Part model, mm, in its own coordinate system. A direction names the side the tool comes from. Round coordinates to 2 decimals unless told otherwise and drop trailing zeros. Order: outer loops, then holes, each group sorted by start corner. A loop starts at its lowest first (then second) coordinate and runs counter-clockwise, first axis right, second up. Notation, with made-up numbers: (-3.5, 75.5) - (22.5, 75.5) arc R26 ccw to (22.5, 97.5) - close; hole circle Ø1 at (-37, 52.5). An arc over 180 degrees is marked (long way). Answer as a JSON object with one key per item and string values.
Autodesk Inventor part; units mm, degrees
ref_plane "YZ Plane" through (0, 0, 0) normal (1, 0, 0) x (0, 1, 0)
ref_plane "XZ Plane" through (0, 0, 0) normal (0, 1, 0) x (-1, 0, 0)
ref_plane "XY Plane" through (0, 0, 0) normal (0, 0, 1) x (1, 0, 0)
sketch "Skizze1" plane through (0, 0, 0) normal (0, 0, 1) x (1, 0, 0)
  line L0 (0.6661, 17.7191) -> (-7.3339, 17.7191)
  line L1 (-7.3339, 17.7191) -> (-7.3339, -8.6809)
  line L2 (-7.3339, -8.6809) -> (18.6661, -8.6809)
  line L3 (18.6661, -8.6809) -> (18.6661, -4.6809)
  line L4 (18.6661, -4.6809) -> (-3.3339, -4.6809)
  line L5 (-3.3339, -4.6809) -> (-3.3339, 13.7191)
  line L6 (-3.3339, 13.7191) -> (0.6661, 13.7191)
  line L7 (0.6661, 13.7191) -> (0.6661, 17.7191)
  circle A0 centre (-5.3339, 15.7191) radius 0.5
  circle A1 centre (-5.3339, -6.6809) radius 0.5
  circle A2 centre (16.6661, -6.6809) radius 0.5
  point P0 (0, 0)
  point P1 (18.6661, -6.6809)
  point P2 (-1.3339, 13.7191)
  dimension "d0" = 26
  dimension "d1" = 26.4
  dimension "d2" = 4
  dimension "d3" = 4
  dimension "d4" = 4
  dimension "d5" = 4
  dimension "d6" = 1
  dimension "d7" = 1
  dimension "d8" = 1
  dimension "d9" = 2
  dimension "d10" = 2
  dimension "d11" = 2
  dimension "d12" = 2
  dimension "d13" = 2
  dimension "d14" = 2
extrude "Extrusion1" add sketch "Skizze1" along normal blind 4.8 contours L7 L6 L5 L4 L3 L2 L1 L0 | A0 | A1 | A2
extrude "Extrusion2" add sketch "Skizze1" along normal blind 5.7 contours A0 | A1 | A2
chamfer "Fase1" distance 0.2 angle 45 1 edges at (-5.8339, 15.7191, 5.7)
chamfer "Fase2" distance 0.2 angle 45 2 edges at (-5.8339, -6.6809, 5.7) (16.1661, -6.6809, 5.7)
sketch "Skizze2" plane through (-7.3339, -8.6809, 0) normal (0, -1, 0) x (1, 0, 0)
  line L0 (5, 5.5045) -> (21, 5.5045)
  line L1 (21, 5.5045) -> (21, 3.8)
  line L2 (21, 3.8) -> (5, 3.8)
  line L3 (5, 3.8) -> (5, 5.5045)
  line L4 (0, 0) -> (0, 4.8)
  line L5 (26, 0) -> (26, 4.8)
  line L6 (0, 4.8) -> (26, 4.8)
  line L7 (11.1841, -1.1388) -> (15.6513, -1.1388)
  line L8 (15.6513, -1.1388) -> (15.6513, 1.113)
  line L9 (15.6513, 1.113) -> (11.1841, 1.113)
  line L10 (11.1841, 1.113) -> (11.1841, -1.1388)
  point P0 (7.3339, 0)
  point P1 (21, 4.6522)
  dimension "d25" = 16
  dimension "d26" = 26
  dimension "d27" = 5
  dimension "d28" = 1
extrude "Extrusion3" cut sketch "Skizze2" against normal blind 5.7
sketch "Skizze3" plane through (-7.3339, -8.6809, 0) normal (-1, 0, 0) x (0, 0, 1)
  line L0 (6.3376, 19.9761) -> (2.8, 19.9761)
  line L1 (2.8, 19.9761) -> (2.8, 12.567)
  line L2 (2.8, 12.567) -> (6.3376, 12.567)
  line L3 (6.3376, 12.567) -> (6.3376, 19.9761)
  line L4 (-2.0066, 6.6289) -> (1.5, 6.6289)
  line L5 (1.5, 6.6289) -> (1.5, 14.728)
  line L6 (1.5, 14.728) -> (-2.0066, 14.728)
  line L7 (-2.0066, 14.728) -> (-2.0066, 6.6289)
  line L8 (4.8, 26.4) -> (4.8, 0)
  line L9 (0, 26.4) -> (0, 0)
  point P0 (0, 8.6809)
  dimension "d33" = 2
  dimension "d34" = 1.5
extrude "Extrusion4" cut sketch "Skizze3" against normal blind 5.7
fillet "Rundung1" radius 1 1 edges at (18.6661, -8.6809, 2.4)
fillet "Rundung2" radius 1 5 edges at (0.6661, 13.7191, 2.4) (18.6661, -4.6809, 2.4) (0.6661, 17.7191, 2.4) (-7.3339, -8.6809, 2.4) (-7.3339, 17.7191, 2.4)
sketch "Skizze4" plane through (-7.3339, -2.052, 1.5) normal (-1, 0, 0) x (0, 0, 1)
  line L0 (-1.5, 8.0991) -> (-1.5, 15.7711)
  line L1 (-1.5, 14.5578) -> (0.4295, 14.5578)
  line L2 (0.4295, 14.5578) -> (0.4295, 17.4567)
  line L3 (0.4295, 17.4567) -> (-1.5, 17.4567)
  line L4 (-1.5, 17.4567) -> (-1.5, 14.5578)
  point P0 (-1.5, 2.052)
  point P1 (-1.5, 15.7711)
extrude "Extrusion5" cut sketch "Skizze4" against normal blind 10
equation "\"d3\" = d2"
equation "\"d5\" = d4"
equation "\"d7\" = d6"
equation "\"d8\" = d6"
equation "\"d9\" = 0.5 * d4"
equation "\"d10\" = d9"
equation "\"d11\" = d10"
equation "\"d12\" = d10"
equation "\"d13\" = d11"
equation "\"d14\" = d13"
properties part number "DisplayUnterlage"
Item 1: Two-plate mould, pull along X, no slides. Class faces 5 (the flat face through (6, -7, 3.8)), 6 (the cylindrical face through (-4.857, 15.569, 5.145)), 7 (the cylindrical face through (0.365, 14.004, 3.385)): pulls with the +X half, pulls with the -X half, needs draft (parallel to the pull), parting line crosses it, or undercut.
Taken from the geometry:
{"face 5": "undercut", "face 6": "parting line crosses it", "face 7": "pulls with the +X half"}
Item 2: Cut at A-A (z = 0.6). Write the cut outline in (x, y).
Taken from the geometry:
{"outline": "(-7.33, -7.68) arc R1 ccw to (-6.33, -8.68) - (3.85, -8.68) - (3.85, -4.68) - (-3.33, -4.68) - (-3.33, -2.05) - (-7.33, -2.05) - close; (-7.33, 6.05) - (-3.33, 6.05) - (-3.33, 12.51) - (-7.33, 12.51) - close; (-7.33, 15.4) - (0.67, 15.4) - (0.67, 16.72) arc R1 ccw to (-0.33, 17.72) - (-6.33, 17.72) arc R1 ccw to (-7.33, 16.72) - close; (8.32, -8.68) - (17.67, -8.68) arc R1 ccw to (18.67, -7.68) - (18.67, -5.68) arc R1 ccw to (17.67, -4.68) - (8.32, -4.68) - close"}
Item 3: Drop flat-ended pins along their axis: P1, Ø3, axis at y = 13, z = 1, coming from the +X side; P2, Ø2, axis at x = 6.5, y = -6.5, coming from the -Z side; P3, Ø3, axis at x = 7.5, y = -5.5, coming from the +Z side. Give the stop position or say it passes through.
Taken from the geometry:
{"P1": "x = 0.51", "P2": "z = 1.11", "P3": "z = 3.8"}
Item 4: Cut at B-B (z = 3.35). Write the cut outline in (x, y).
Taken from the geometry:
{"outline": "(-7.33, -7.68) arc R1 ccw to (-6.33, -8.68) - (17.67, -8.68) arc R1 ccw to (18.67, -7.68) - (18.67, -5.68) arc R1 ccw to (17.67, -4.68) - (-3.33, -4.68) - (-3.33, 3.89) - (-7.33, 3.89) - close; (-7.33, 11.3) - (-3.33, 11.3) - (-3.33, 13.72) - (-0.33, 13.72) arc R1 ccw to (0.67, 14.72) - (0.67, 16.72) arc R1 ccw to (-0.33, 17.72) - (-6.33, 17.72) arc R1 ccw to (-7.33, 16.72) - close"}
Item 5: Tool access for faces 1 (the cylindrical face through (16.167, -6.703, 5.145)), 2 (the flat face through (-5, 6.047, 1)), 3 (the flat face through (8.317, -6.7, 0.5)), 4 (the flat face through (7, -4.681, 2)): list every direction of +Z, -Z, +X, -X, +Y, -Y with a clear straight run to the whole face (end or side of a thin tool).
Taken from the geometry:
{"face 1": "+Z", "face 2": "-Z, +X, -X", "face 3": "-Z, +Y, -Y", "face 4": "+Z, -Z, +X"}
Item 6: Cut at C-C (y = 3). Write the cut outline in (x, z), plus the area to 3 significant figures.
Taken from the geometry:
{"outline": "(-7.33, 1.5) - (-3.33, 1.5) - (-3.33, 4.8) - (-7.33, 4.8) - close", "area": "13.2 mm2"}
Item 7: Cut at D-D (x = 1). Write the cut outline in (y, z).
Taken from the geometry:
{"outline": "(-8.68, 0) - (-4.68, 0) - (-4.68, 3.8) - (-8.68, 3.8) - close"}
Item 8: Probe L1, parallel to Y at x = -6, z = 1.15; L2, parallel to Y at x = -3.25, z = 1.65; L3, parallel to X at y = -0.75, z = 4.15. List the from-to ranges inside material, lowest first. Write a range as from..to.
Taken from the geometry:
{"L1": "-8.68..-2.05, 6.05..12.51, 15.4..17.72", "L2": "-8.68..-4.68, 15.4..17.72", "L3": "-7.33..-3.33"}
